Check sheet for the modelled part. Datum: model origin and axes. Units: mm. Face numbers are marked on the shaded views. A direction names the side the tool comes from. Round coordinates to 2 decimals unless told otherwise and drop trailing zeros. Loops run counter-clockwise (first coordinate to the right, second up) from the corner with the lowest first, then second, coordinate; pieces in that order, holes last. Notation, with made-up numbers: (13.5, -38) -> (19.5, -38) arc R30 ccw to (19.5, -14) -> close; hole circle Ø7 at (-10, 56.5). An arc over 180 degrees is marked (long way). Use one line per item in the form item = value. Start each with the question number.
(1) Draft check along X on the marked faces 4, 5 and 6. Enter one of: released by +X, released by -X, zero draft, split by the parting line, or undercut.
(2) Sectioned sample at C-C (y = -15). Record the cut outline in (x, z).
(3) Material ranges on probe 1 along Y at (x, z) = (0, 5.75); probe 2 along Z at (x, y) = (4, 16.5); probe 3 along Z at (x, y) = (14, 9.5), recorded low to high. Write a range as [from, to].
(4) Set-up check for the marked faces 1, 2 and 3: record each of +Z, -Z, +X, -X, +Y, -Y from which the full face is reachable in a straight line by a thin tool's end or side.
(5) Go/stop test with flat-tipped pins: pin 1 (1.5 mm diameter, centred on x = -1, y = 3, fed in from -Z); pin 2 (4 mm diameter, centred on x = -6, y = -14, fed in from +Z); pin 3 (8 mm diameter, centred on x = -1.5, z = 30, fed in from +Y). Record where each tip stops, or that it passes through.
(6) Sectioned sample at A-A (y = 15). Record the cut outline in (x, z), and give its area (3 significant figures).
(7) Sectioned sample at B-B (x = 0). Record the cut outline in (y, z), and give its area (3 significant figures).
from build123d import *

# Parameters (mm, degrees)
SKETCH1_W           = 42
SKETCH1_H           = 42
BOSS_EXTRUDE1_DEPTH = 95.2
SKETCH2_R           = 11
BOSS_EXTRUDE2_DEPTH = 22
SKETCH3_W           = 15.8
SKETCH3_H           = 27.7
CUT_EXTRUDE1_DEPTH  = 21
SKETCH4_R           = 5
CUT_EXTRUDE2_DEPTH  = 10
CHAMFER1_SIZE       = 3
FILLET1_R           = 3
FILLET2_R           = 1


with BuildPart() as part:
    # Sketch1 → Boss-Extrude1 (new body)
    with BuildSketch(Plane.XY):
        Rectangle(SKETCH1_W, SKETCH1_H)
    extrude(amount=BOSS_EXTRUDE1_DEPTH)

    # Sketch2 → Boss-Extrude2 (add)
    with BuildSketch(Plane.XY.offset(95.2)):
        with Locations((0, 0.393132524)):
            Circle(SKETCH2_R)
    extrude(amount=BOSS_EXTRUDE2_DEPTH)

    # Sketch3 → Cut-Extrude1 (cut)
    with BuildSketch(Plane(origin=(0, 21, 0), x_dir=(1, 0, 0), z_dir=(0, 1, 0))):
        with Locations((0, -33.35)):
            Rectangle(SKETCH3_W, SKETCH3_H)
    extrude(amount=-CUT_EXTRUDE1_DEPTH, mode=Mode.SUBTRACT)

    # Sketch4 → Cut-Extrude2 (cut)
    with BuildSketch(Plane(origin=(0, 0, 0), x_dir=(-1, 0, 0), z_dir=(0, 0, -1))):
        Circle(SKETCH4_R)
    extrude(amount=-CUT_EXTRUDE2_DEPTH, mode=Mode.SUBTRACT)

    # Chamfer1
    chamfer1_edges = [part.edges().sort_by_distance(p)[0] for p in [
        (21, -21, 47.6),
        (-21, -21, 47.6),
        (-21, 21, 47.6),
        (21, 21, 47.6),
    ]]
    chamfer(chamfer1_edges, length=CHAMFER1_SIZE)

    # Fillet1
    # the kernel refuses this fillet: 3 mm, written as the material it takes off along each edge
    with BuildSketch(Plane(origin=(-21, 25.5, 95.2), x_dir=(1, 0, 0), z_dir=(0, -1, 0)), Plane(origin=(21, -25.5, 95.2), x_dir=(-1, 0, 0), z_dir=(0, 1, 0)), Plane(origin=(25.5, 21, 95.2), x_dir=(0, -1, 0), z_dir=(-1, 0, 0))) as fillet1_piece_1:
        with BuildLine():
            CenterArc((FILLET1_R, -FILLET1_R), FILLET1_R, 90, 90)
            Line((0, -FILLET1_R), (0, 0))
            Line((0, 0), (FILLET1_R, 0))
        make_face()
    extrude(amount=51, mode=Mode.SUBTRACT)
    with BuildSketch(Plane(origin=(-25.5, -21, 95.2), x_dir=(0, 0, -1), z_dir=(1, 0, 0))) as fillet1_piece_2:
        with BuildLine():
            CenterArc((FILLET1_R, FILLET1_R), FILLET1_R, 180, 90)
            Line((0, FILLET1_R), (0, 0))
            Line((0, 0), (FILLET1_R, 0))
        make_face()
    extrude(amount=51, mode=Mode.SUBTRACT)

    # Fillet2
    fillet2_edges = [part.edges().sort_by_distance(p)[0] for p in [
        (-11, 0.393132524, 117.2),
    ]]
    fillet(fillet2_edges, radius=FILLET2_R)


solid = part.part
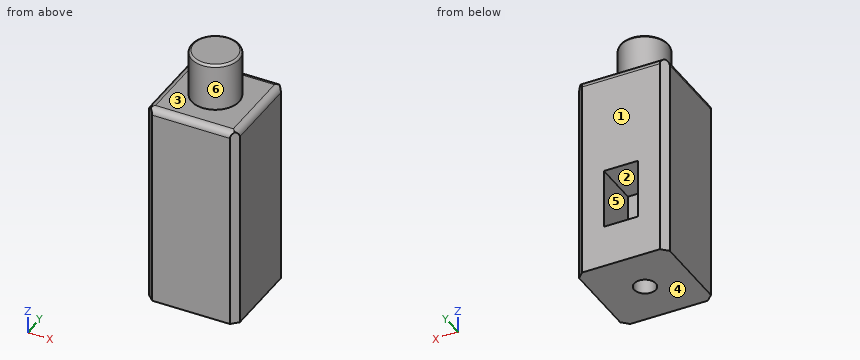
Checks:
q1.face_4 = zero draft
q1.face_5 = undercut
q1.face_6 = split by the parting line
q2.outline = (-21, 0) -> (21, 0) -> (21, 92.2) arc R3 ccw to (18, 95.2) -> (-18, 95.2) arc R3 ccw to (-21, 92.2) -> close
q3.probe_1 = [-21, -5], [5, 21]
q3.probe_2 = [0, 19.5], [47.2, 95.2]
q3.probe_3 = [0, 95.2]
q4.face_1 = +Z, -Z, +X, -X, +Y
q4.face_2 = +Y
q4.face_3 = +Z
q5.pin_1 = 10
q5.pin_2 = 95.2
q5.pin_3 = 0
q6.outline = (-21, 0) -> (21, 0) -> (21, 92.2) arc R3 ccw to (18, 95.2) -> (-18, 95.2) arc R3 ccw to (-21, 92.2) -> close; hole (-7.9, 19.5) -> (7.9, 19.5) -> (7.9, 47.2) -> (-7.9, 47.2) -> close
q6.area = 3,560 mm2
q7.outline = (-21, 0) -> (-5, 0) -> (-5, 10) -> (5, 10) -> (5, 0) -> (21, 0) -> (21, 19.5) -> (0, 19.5) -> (0, 47.2) -> (21, 47.2) -> (21, 92.2) arc R3 ccw to (18, 95.2) -> (11.39, 95.2) -> (11.39, 116.2) arc R1 ccw to (10.39, 117.2) -> (-9.61, 117.2) arc R1 ccw to (-10.61, 116.2) -> (-10.61, 95.2) -> (-18, 95.2) arc R3 ccw to (-21, 92.2) -> close
q7.area = 3,800 mm2
